Autodesk Fusion 360 part; units mm, degrees
sketch "Sketch1" plane through (0, 0, 0) normal (0, 0, 1) x (1, 0, 0)
  circle A0 centre (0, 0) radius 38.1
  circle A1 centre (0, 0) radius 36.1
  line L0 (23.3872, -27.5) -> (23.3872, 27.5)
  line L1 (25.3872, -25.6652) -> (25.3872, 25.6652)
  line L2 (25.3872, 12.5) -> (27.3872, 12.5)
  line L3 (27.3872, 12.5) -> (27.3872, -12.5)
  line L4 (27.3872, -12.5) -> (25.3872, -12.5)
  line L5 (25.3872, -12.5) -> (25.3872, 12.5)
  line L6 (25.3872, 14.5) -> (29.3872, 14.5)
  line L7 (29.3872, 14.5) -> (29.3872, 9.5)
  line L8 (29.3872, 9.5) -> (27.3872, 9.5)
  line L9 (25.3872, -14.5) -> (29.3872, -14.5)
  line L10 (29.3872, -14.5) -> (29.3872, -9.5)
  line L11 (29.3872, -9.5) -> (27.3872, -9.5)
  line L12 (1.75, 0) -> (22.5, 0)
  line L13 (23.3872, 26.75) -> (20.8872, 26.75)
  line L14 (20.8872, 26.75) -> (20.8872, -26.75)
  line L15 (20.8872, -26.75) -> (23.3872, -26.75)
  line L16 (23.3872, -26.75) -> (23.3872, 26.75)
  line L17 (20.8872, 18.08) -> (8.8872, 18.08)
  line L18 (8.8872, 18.08) -> (8.8872, 5.08)
  line L19 (8.8872, 5.08) -> (20.8872, 5.08)
  line L20 (20.8872, 5.08) -> (20.8872, 18.08)
  line L21 (20.8872, -12.5) -> (8.8872, -12.5)
  line L22 (8.8872, -12.5) -> (8.8872, -22.5)
  line L23 (8.8872, -22.5) -> (20.8872, -22.5)
  line L24 (20.8872, -22.5) -> (20.8872, -12.5)
  line L25 (29.3872, -9.5) -> (29.3872, 9.5)
  line L26 (0, -38.1) -> (0, 38.1) construction
  line L27 (-38.1, 0) -> (38.1, 0) construction
  line L28 (26.9408, -26.9408) -> (-26.9408, 26.9408) construction
  line L29 (26.9408, 26.9408) -> (-26.9408, -26.9408) construction
  line L30 (0, 36.1) -> (0, 38.1)
  line L31 (-25.5266, 25.5266) -> (-26.9408, 26.9408)
  line L32 (-36.1, 0) -> (-38.1, 0)
  line L33 (-26.9408, -26.9408) -> (-25.5266, -25.5266)
  line L34 (0, -38.1) -> (0, -36.1)
  line L35 (26.9408, -26.9408) -> (25.5266, -25.5266)
  line L36 (38.1, 0) -> (36.1, 0)
  line L37 (26.9408, 26.9408) -> (25.5266, 25.5266)
  line L38 (18.8872, 30.765) -> (18.8872, 20.08)
  line L39 (18.8872, 20.08) -> (6.8872, 20.08)
  line L40 (6.8872, 20.08) -> (6.8872, 3.08)
  line L41 (6.8872, 3.08) -> (20.8872, 3.08)
  line L42 (-37.7705, 5) -> (-35.7705, 5)
  line L43 (-35.7705, 5) -> (-35.7705, -5)
  line L44 (-35.7705, -5) -> (-37.7705, -5)
  line L45 (-37.7705, -5) -> (-37.7705, 5)
  line L46 (-12.7705, 5) -> (-10.7705, 5)
  line L47 (-10.7705, 5) -> (-10.7705, -5)
  line L48 (-10.7705, -5) -> (-12.7705, -5)
  line L49 (-12.7705, -5) -> (-12.7705, 5)
  line L50 (-29.2705, 24) -> (-19.2705, 24)
  line L51 (-19.2705, 24) -> (-19.2705, 22)
  line L52 (-19.2705, 22) -> (-29.2705, 22)
  line L53 (-29.2705, 22) -> (-29.2705, 24)
  line L54 (-29.2705, -22) -> (-19.2705, -22)
  line L55 (-19.2705, -22) -> (-19.2705, -24)
  line L56 (-19.2705, -24) -> (-29.2705, -24)
  line L57 (-29.2705, -24) -> (-29.2705, -22)
  line L58 (-25.7705, 16.5) -> (-17.7705, 16.5)
  line L59 (-17.7705, 16.5) -> (-17.7705, 0.5)
  line L60 (-17.7705, 0.5) -> (-25.7705, 0.5)
  line L61 (-25.7705, 0.5) -> (-25.7705, 16.5)
  point P0 (27.3872, 0)
  point P1 (20.8872, 0)
  point P2 (-33.5, 0)
  point P3 (-20, 24)
  point P4 (-35.7705, 0)
  point P5 (-24.2705, 0)
  point P6 (-24.2705, 22)
  dimension "d1" = 76.2
  dimension "d2" = 2
  dimension "d3" = 55
  dimension "d4" = 2
  dimension "d5" = 2
  dimension "d6" = 2
  dimension "d7" = 2
  dimension "d8" = 3
  dimension "d9" = 25
  dimension "d10" = 2
  dimension "d11" = 2.5
  dimension "d12" = 53.5
  dimension "d13" = 13
  dimension "d14" = 12
  dimension "d15" = 8.67
  dimension "d16" = 10
  dimension "d17" = 12
  dimension "d18" = 4.25
  dimension "d23" = 45
  dimension "d27" = 2
  dimension "d28" = 2
  dimension "d29" = 2
  dimension "d30" = 2
  dimension "d45" = 10
  dimension "d46" = 2
  dimension "d47" = 11.5
  dimension "d48" = 11.5
  dimension "d49" = 22
  dimension "d50" = 22
  dimension "d51" = 16
  dimension "d52" = 8
  dimension "d53" = 1.5
  dimension "d54" = 5.5
extrude "Extrude1" add sketch "Sketch1" along normal blind 2 contours A0 A1 L36 L37 | A0 A1 L35 L36 | A0 A1 L30 L37 | A0 A1 L34 L35 | A1 L1 L6 L7 L9 L10 L25 | A0 A1 L30 L31 | A0 A1 L33 L34 | A0 A1 L31 L42 L43 L50 L52 L53 | A1 L0 L14 L15 L21 L22 L23 L38 L39 L40 L41 L43 L50 L51 L52 L54 L55 L56 | A0 A1 L33 L43 L44 L54 L56 L57 | A0 L32 L45 | A1 L32 L42 L43 L45 | A1 L0 L13 L14 L17 L18 L19 L38 L39 L40 L41 | A1 L32 L43 L44 L45 | A0 L32 L45 | A1 L50 L51 L52 | A1 L50 L52 L53 | L0 L13 L14 L15 L16 L20 L24 | A1 L54 L56 L57 | A1 L54 L55 L56 | A1 L43 | L46 L47 L48 L49
extrude "Extrude4" add sketch "Sketch1" along normal blind 10 contours A1 L0 L13 L14 L17 L18 L19 L38 L39 L40 L41
extrude "Extrude6" add sketch "Sketch1" along normal blind 50 contours A1 L0 L1 L5 L16
extrude "Extrude7" add sketch "Sketch1" along normal blind 15 contours A1 L32 L42 L43 L45 | L1 L2 L3 L6 L7 L8 | A1 L32 L43 L44 L45 | L1 L3 L4 L9 L10 L11 | A1 L50 L51 L52 | A1 L50 L52 L53 | A1 L54 L56 L57 | A1 L54 L55 L56 | A1 L43 | L46 L47 L48 L49
equation "d47 = ( 23 / 2 ) * 1 mm"
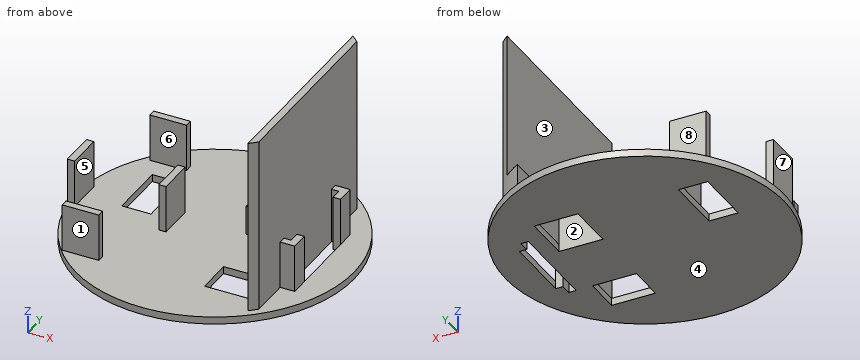
Work out the finished part from the listing and answer in its coordinate system (mm). Face numbers are marked on the shaded views. A direction names the side the tool comes from. Give positions to 0.01 mm unless a question says otherwise; leave off trailing zeros. Write each loop counter-clockwise with the first axis right and the second up, starting at its lowest first coordinate (ties: lowest second). Pieces come first, ordered by that corner, then holes. Notation, with made-up numbers: M 10,-21.5 L 67,-21.5 A24 ccw 67,-1.5 Z; hole C 88.5,-18 d11. An arc over 180 degrees is marked long. Answer as CSV lines item,"result".
Q1. A cutting plane is placed at A-A on y = -11. Write down the section's boundary in (x, z).
A:
outline,"M -36.48,0 L 25.39,0 L 25.39,50 L 23.39,50 L 23.39,2 L -36.48,2 Z; M 27.39,0 L 36.48,0 L 36.48,2 L 29.39,2 L 29.39,15 L 27.39,15 Z"
Q2. Given P1, Ø2, axis at x = -20, z = 1, coming from the +Y side; P2, Ø1.6, axis at y = 23, z = 11.5, coming from the +X side; P3, Ø8, axis at x = 12.5, y = 5.5, coming from the +Z side; P4, Ø3, axis at x = 26.5, y = -13, coming from the +Z side, each flat-ended and moving along its own axis, determine where each tip first touches the part or whether it passes through.
A:
P1,"stops at y = 33.02"
P2,"stops at x = 25.39"
P3,"stops at z = 10"
P4,"stops at z = 50"
Q3. The mould has two halves that part along Y. Classify the marked faces 1, 2 and 3: +Y half, -Y half, draft (parallel to the pull), parting line (faces both ways), or undercut.
A:
face 1,"-Y half"
face 2,"undercut"
face 3,"draft"
Q4. A cutting plane is placed at C-C on y = 6.5. Write down the section's boundary in (x, z).
A:
outline,"M -37.54,0 L -25.77,0 L -25.77,2 L -37.54,2 Z; M -17.77,0 L 8.89,0 L 8.89,10 L 6.89,10 L 6.89,2 L -17.77,2 Z; M 20.89,0 L 25.39,0 L 25.39,50 L 23.39,50 L 23.39,2 L 20.89,2 Z; M 29.39,0 L 37.54,0 L 37.54,2 L 29.39,2 Z"
Q5. A tool of negligible diameter and unlimited length cuts with its end or side. For the marked faces 4, 5, 6, 7 and 8, from which of +Z, -Z, +X, -X, +Y, -Y can it reach the whole face along a straight path? Write none if from no direction.
A:
face 4,"-Z, +X, -X, +Y, -Y"
face 5,"+Z, +Y, -Y"
face 6,"+Z, -X"
face 7,"+Z, -X, +Y, -Y"
face 8,"+Z, -X, +Y"
Q6. A cutting plane is placed at B-B on x = 12. Write down the section's boundary in (y, z).
A:
outline,"M -36.16,0 L -22.5,0 L -22.5,2 L -36.16,2 Z; M -12.5,0 L 5.08,0 L 5.08,10 L 3.08,10 L 3.08,2 L -12.5,2 Z; M 18.08,0 L 36.16,0 L 36.16,2 L 20.08,2 L 20.08,10 L 18.08,10 Z"
Q7. A cutting plane is placed at D-D on x = 0. Write down the section's boundary in (y, z), plus the area to 3 significant figures.
A:
outline,"M -38.1,0 L 38.1,0 L 38.1,2 L -38.1,2 Z"
area,"152 mm²"
Q8. Find the intervals of material crossed by probe 1 along X at (y, z) = (-12, 12.5); probe 2 along X at (y, z) = (17.5, 9.5); probe 3 along Z at (x, y) = (6, 9), in increasing order. Write a range as [from, to].
A:
probe 1,"x = [23.39, 25.39], [27.39, 29.39]"
probe 2,"x = [6.89, 8.89], [23.39, 25.39]"
probe 3,"z = [0, 2]"
